Answer from the drawing. Dimensions are ordinates in mm from the lowest x, y and z of the part. A direction names the side the tool comes from. Give positions to 0.01 mm unless a question says otherwise; leave off trailing zeros. Loops run counter-clockwise (first coordinate to the right, second up) from the corner with the lowest first, then second, coordinate; pieces in that order, holes last.
Item 1: Section C-C, the plane y = 5.5 is taken. Give the vertices of the cut face in (x, z).
Item 2: Consider line 1 along Z through (x, y) = (10, 5.75); line 2 along Y through (x, z) = (11.35, 0.6) (3 decimals); line 3 along X through (y, z) = (3.25, 3). Determine where each line is inside the solid, lowest interval first.
Item 3: A tool of negligible diameter and unlimited length cuts with its end or side. For the marked faces 4, 5 and 6, from which of +Z, -Z, +X, -X, +Y, -Y can it reach the whole face along a straight path? Write none if from no direction.
Item 4: Section D-D, the plane y = 8.5 is taken. Give the vertices of the cut face in (x, z) (3 decimals).
Item 5: Each of these flat-tipped pins is pushed along its axis until it touches: pin 1 Ø5.5 at (x, y) = (20.5, 6.5) entering from -Z; pin 2 Ø1 at (y, z) = (2.5, 6) entering from -X; pin 3 Ø1 at (x, y) = (5.5, 6.5) entering from +Z; pin 4 Ø6 at (x, z) = (21.5, 5) entering from -Y. Where does it stop, or does it pass through?
Item 6: Section B-B, the plane x = 21.35 is taken. Give the vertices of the cut face in (y, z) (3 decimals), and give its area (3 significant figures).
Item 7: Section A-A, the plane z = 3.5 is taken. Give the vertices of the cut face in (x, y).
Item 8: The mould has two halves that part along X. Classify the marked faces 1, 2 and 3: pulls with the +X half, pulls with the -X half, needs draft (parallel to the pull), parting line crosses it, or undercut.
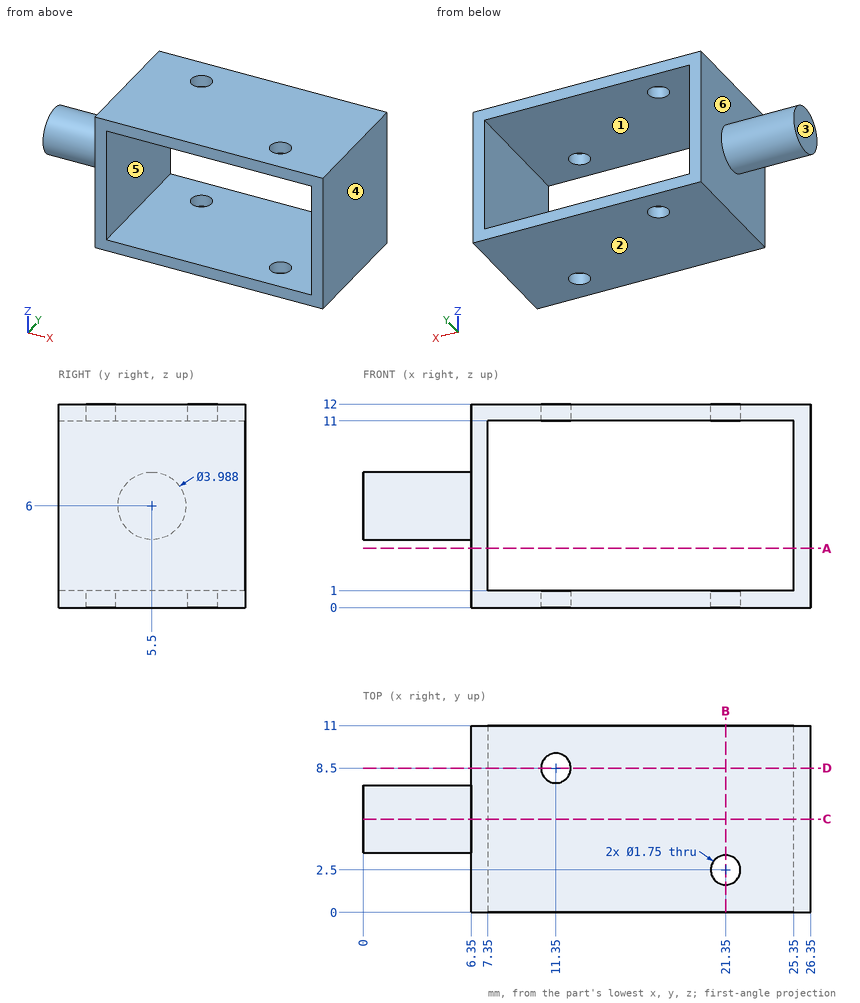
Worked answers:
1. outline: (0, 4.01) - (6.35, 4.01) - (6.35, 0) - (26.35, 0) - (26.35, 12) - (6.35, 12) - (6.35, 7.99) - (0, 7.99) - close; hole (7.35, 1) - (25.35, 1) - (25.35, 11) - (7.35, 11) - close
2. line 1: z = 0 to 1, 11 to 12
2. line 2: y = 0 to 7.625, 9.375 to 11
2. line 3: x = 6.35 to 7.35, 25.35 to 26.35
3. face 4: +Z, -Z, +X, +Y, -Y
3. face 5: +Y, -Y
3. face 6: -X
4. outline: (6.35, 0) - (10.475, 0) - (10.475, 1) - (7.35, 1) - (7.35, 11) - (10.475, 11) - (10.475, 12) - (6.35, 12) - close; (12.225, 0) - (26.35, 0) - (26.35, 12) - (12.225, 12) - (12.225, 11) - (25.35, 11) - (25.35, 1) - (12.225, 1) - close
5. pin 1: stops at z = 0
5. pin 2: stops at x = 6.35
5. pin 3: stops at z = 7.93
5. pin 4: passes through
6. outline: (0, 0) - (1.625, 0) - (1.625, 1) - (0, 1) - close; (0, 11) - (1.625, 11) - (1.625, 12) - (0, 12) - close; (3.375, 0) - (11, 0) - (11, 1) - (3.375, 1) - close; (3.375, 11) - (11, 11) - (11, 12) - (3.375, 12) - close
6. area: 18.5 mm2
7. outline: (6.35, 0) - (7.35, 0) - (7.35, 11) - (6.35, 11) - close; (25.35, 0) - (26.35, 0) - (26.35, 11) - (25.35, 11) - close
8. face 1: undercut
8. face 2: needs draft
8. face 3: pulls with the -X half
